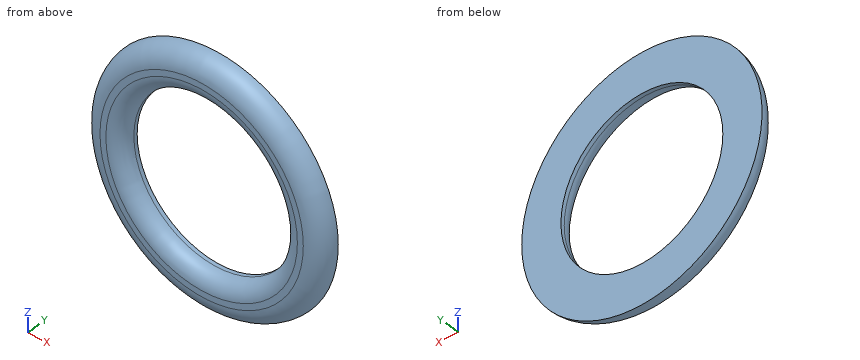
```python
from build123d import *

# Parameters (mm, degrees)
F0_R     = 3.25
F0_R_2   = 2.19
F1_DEPTH = 0.5
F2_R     = 0.49999
F3_R     = 0.4


# Not quite as in the source:
# - a fillet or chamfer is up to 0.001 mm smaller than in the source, because OpenCascade refuses the exact size


with BuildPart() as f1:
    # F0 (on Front) → F1 (new body)
    with BuildSketch(Plane.XZ):
        Circle(F0_R)
        Circle(F0_R_2, mode=Mode.SUBTRACT)
    extrude(amount=F1_DEPTH)

    # F2 (radius 0.5 in the source; OpenCascade refuses exactly that, so slightly less here)
    f2_edges = [f1.edges().sort_by_distance(p)[0] for p in [
        (-3.25, -0.5, 0),
    ]]
    fillet(f2_edges, radius=F2_R)

    # F3
    f3_edges = [f1.edges().sort_by_distance(p)[0] for p in [
        (-2.19, -0.5, 0),
    ]]
    fillet(f3_edges, radius=F3_R)


solid = f1.part
```
Geometry check sheet. Reference: the model listing, model coordinates, mm. Coordinates: 2 decimals unless noted, no trailing zeros. Write each loop counter-clockwise with the first axis right and the second up, starting at its lowest first coordinate (ties: lowest second). Pieces come first, ordered by that corner, then holes. Notation, with made-up numbers: M 56,86 L 82,86 A20 ccw 82,103 Z; hole C 41,-7.5 d11. An arc over 180 degrees is marked long. One line per item, written item: value. Start each with the question number.
(1) Sectioned sample at C-C, the plane y = -0.25. Enter the section's corners in (x, z).
(2) Depth check by flat-ended pin: pin 1 (2.5 mm diameter, centred on x = 0, z = 0, fed in from +Y). Enter the tip coordinate at first touch or a pass-through.
(3) Scan lines: line 1 along X through (y, z) = (-0.3, -1.75); line 2 along Z through (x, y) = (1.25, -0.4); line 3 along Z through (x, y) = (-1.25, -0.2). Record each from-to range of solid material in increasing order. Write a range as [from, to].
Filled sheet:
1. outline: C 0,0 d6.37; hole C 0,0 d4.44
2. pin 1: through
3. line 1: [-2.62, -1.4], [1.4, 2.62]
3. line 2: [-2.78, -1.96], [1.96, 2.78]
3. line 3: [-2.95, -1.81], [1.81, 2.95]
